Here's the drawing with two shaded views (mm, measured from the low corner). I have some questions. A direction names the side the tool comes from. Coordinates: 2 decimals unless noted, no trailing zeros. Loops run counter-clockwise (first coordinate to the right, second up) from the corner with the lowest first, then second, coordinate; pieces in that order, holes last. Notation, with made-up numbers: M 54.5,58 L 64.5,58 A14 cw 64.5,72 Z; hole C 12.5,18 d4. An arc over 180 degrees is marked long. Return JSON: item names as keys, results as strings. Group by question number.
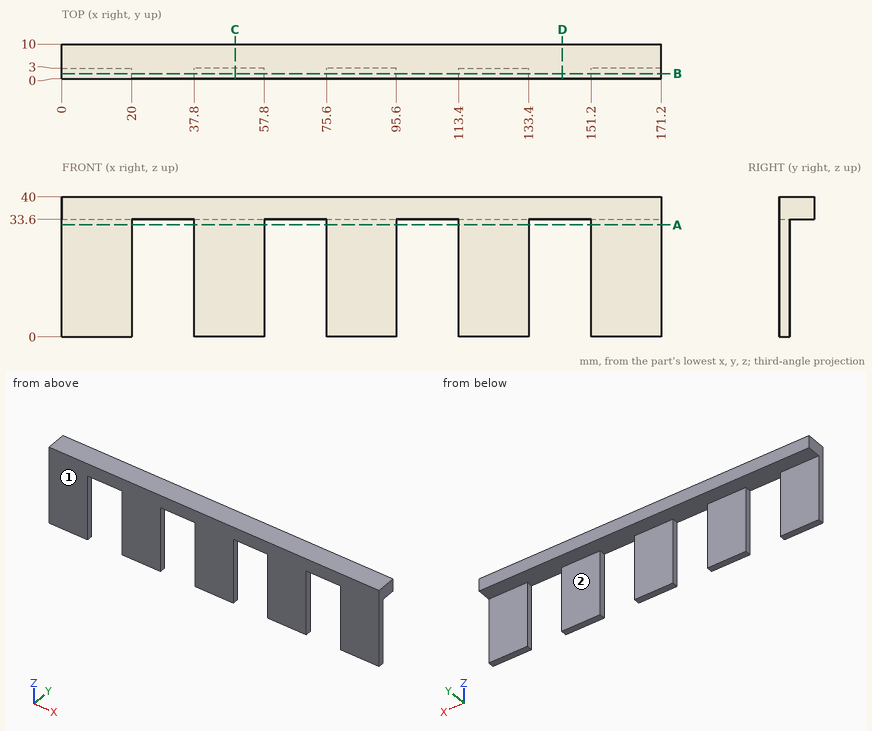
1) If I drill on line 1 (X direction, y = 1.25, z = 8); line 2 (Z direction, x = 29.5, y = 4.75); line 3 (Y direction, x = 153, z = 28.5), over which ranges is the centre line in solid material (lowest first)? Write a range as from..to.
2) Suppose I cut it at B-B, the plane y = 1.5. List the corners of the cut face in (x, z) for me, then the cut area to 3 significant figures.
3) For pin 1 (2.5 mm diameter, centred on y = 1, z = 24, fed in from -X); pin 2 (22 mm diameter, centred on x = 160, z = 13, fed in from +Y); pin 3 (3 mm diameter, centred on x = 126, y = 6.5, fed in from -Z), each with a flat end and sliding along its axis, tell me the tip position at first contact or that it passes through.
4) Suppose I cut it at C-C, the plane x = 49.5. List the corners of the cut face in (y, z) for me.
5) Suppose I cut it at D-D, the plane x = 143. List the corners of the cut face in (y, z) for me, then the cut area to 3 significant figures.
6) Suppose I cut it at A-A, the plane z = 32. List the corners of the cut face in (x, y) for me.
7) For the marked faces 1 and 2, which set-ups out of +Z, -Z, +X, -X, +Y, -Y let a thin tool reach every point of the face, with its end or its side?
Returned:
{
 "1": {"line 1": "x = 0..20, 37.8..57.8, 75.6..95.6, 113.4..133.4, 151.2..171.2", "line 2": "z = 33.6..40", "line 3": "y = 0..3"},
 "2": {"outline": "M 0,0 L 20,0 L 20,33.6 L 37.8,33.6 L 37.8,0 L 57.8,0 L 57.8,33.6 L 75.6,33.6 L 75.6,0 L 95.6,0 L 95.6,33.6 L 113.4,33.6 L 113.4,0 L 133.4,0 L 133.4,33.6 L 151.2,33.6 L 151.2,0 L 171.2,0 L 171.2,40 L 0,40 Z", "area": "4,460 mm²"},
 "3": {"pin 1": "stops at x = 0", "pin 2": "stops at y = 3", "pin 3": "stops at z = 33.6"},
 "4": {"outline": "M 0,0 L 3,0 L 3,33.6 L 10,33.6 L 10,40 L 0,40 Z"},
 "5": {"outline": "M 0,33.6 L 10,33.6 L 10,40 L 0,40 Z", "area": "64.0 mm²"},
 "6": {"outline": "M 0,0 L 20,0 L 20,3 L 0,3 Z; M 37.8,0 L 57.8,0 L 57.8,3 L 37.8,3 Z; M 75.6,0 L 95.6,0 L 95.6,3 L 75.6,3 Z; M 113.4,0 L 133.4,0 L 133.4,3 L 113.4,3 Z; M 151.2,0 L 171.2,0 L 171.2,3 L 151.2,3 Z"},
 "7": {"face 1": "+Z, -Z, +X, -X, -Y", "face 2": "-Z, +X, -X, +Y"}
}
